from build123d import *

# Parameters (mm, degrees)
F0_W        = 130
F0_H        = 130
F1_DEPTH    = 17.5
F2_W        = 126
F2_H        = 31
F3_DEPTH    = 126
F5_W        = 122.3782406645
F5_H        = 23.2565429012
F6_DEPTH    = 7
F4_W        = 119.2743226562
F4_H        = 26.0036256061
F7_DEPTH    = 3
F8_T1_DEPTH = 50


# Not quite as in the source:
# - a fillet or chamfer that OpenCascade refuses, or shapes differently, is made with other operations: its cross-section is extruded or revolved along the edge and cut away or added


with BuildPart() as f1:
    # F0 (on Top) → F1 (new body, symmetric)
    with BuildSketch(Plane.XY):
        with Locations((2.0031377077, 1.1643140912)):
            Rectangle(F0_W, F0_H)
    extrude(amount=F1_DEPTH, both=True)

    # F2 (on face) → F3 (cut)
    with BuildSketch(Plane.XZ.offset(63.8356859088)):
        with Locations((2.0031377077, 0)):
            Rectangle(F2_W, F2_H)
    extrude(amount=-F3_DEPTH, mode=Mode.SUBTRACT)

    # F5 (on face) → F6 (cut)
    with BuildSketch(Plane(origin=(0, 66.1643140912, 0), x_dir=(-1, 0, 0), z_dir=(0, 1, 0))):
        with Locations((-2.0031377077, 0)):
            Rectangle(F5_W, F5_H)
    extrude(amount=-F6_DEPTH, mode=Mode.SUBTRACT)

    # F4 (on face) → F7 (cut)
    with BuildSketch(Plane(origin=(-62.9968622923, 0, 0), x_dir=(0, -1, 0), z_dir=(-1, 0, 0))):
        with Locations((-1.2152138836, -0.0606838628)):
            Rectangle(F4_W, F4_H)
    extrude(amount=-F7_DEPTH, mode=Mode.SUBTRACT)

    # F8: fillet of radius 3 on 4 edges, made by hand

    # F8_s2 → F8_t1 (cut)
    with BuildSketch(Plane.XY.offset(-25)):
        with BuildLine():
            add(Edge.make_bspline(
                [(-59.9968622923, 66.1643140912), (-62.9968622923, 66.1643140912), (-62.9968622923, 63.1643140912)],
                knots=[0, 0, 0, 1, 1, 1], degree=2, weights=[1, 1, 1]))
            Line((-62.9968622923, 63.1643140912), (-62.9968622923, 66.1643140912))
            Line((-62.9968622923, 66.1643140912), (-59.9968622923, 66.1643140912))
        make_face()
        with BuildLine():
            add(Edge.make_bspline(
                [(-62.9968622923, -60.8356859088), (-62.9968622923, -63.8356859088), (-59.9968622923, -63.8356859088)],
                knots=[0, 0, 0, 1, 1, 1], degree=2, weights=[1, 1, 1]))
            Line((-59.9968622923, -63.8356859088), (-62.9968622923, -63.8356859088))
            Line((-62.9968622923, -63.8356859088), (-62.9968622923, -60.8356859088))
        make_face()
        with BuildLine():
            add(Edge.make_bspline(
                [(64.0031377077, 66.1643140912), (67.0031377077, 66.1643140912), (67.0031377077, 63.1643140912)],
                knots=[0, 0, 0, 1, 1, 1], degree=2, weights=[1, 1, 1]))
            Line((67.0031377077, 63.1643140912), (67.0031377077, 66.1643140912))
            Line((67.0031377077, 66.1643140912), (64.0031377077, 66.1643140912))
        make_face()
        with BuildLine():
            add(Edge.make_bspline(
                [(67.0031377077, -60.8356859088), (67.0031377077, -63.8356859088), (64.0031377077, -63.8356859088)],
                knots=[0, 0, 0, 1, 1, 1], degree=2, weights=[1, 1, 1]))
            Line((64.0031377077, -63.8356859088), (67.0031377077, -63.8356859088))
            Line((67.0031377077, -63.8356859088), (67.0031377077, -60.8356859088))
        make_face()
    extrude(amount=F8_T1_DEPTH, mode=Mode.SUBTRACT)


solid = f1.part
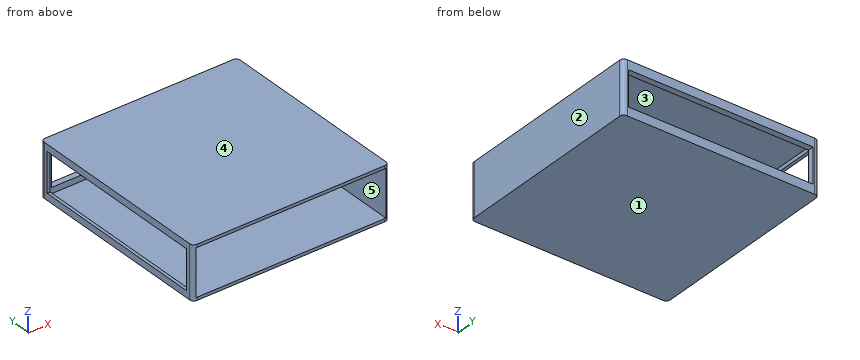
Build history of the part. All positions in model axes, mm. Face numbers are marked on the shaded views. A direction names the side the tool comes from. Round coordinates to 2 decimals unless told otherwise and drop trailing zeros. Loops run counter-clockwise (first coordinate to the right, second up) from the corner with the lowest first, then second, coordinate; pieces in that order, holes last. Notation, with made-up numbers: (67.25, 27.25) -> (108.25, 27.25) arc R19 ccw to (108.25, 44.25) -> close; hole circle Ø4 at (23, 1). An arc over 180 degrees is marked (long way). Use CSV: the item, a comma, the result in double quotes. Start each with the question number.
Q1. Saw through at A-A on x = -44. Give the cut face in (y, z).
Q2. Saw through at B-B on z = -9.5. Count the separate pieces of the cut face and the enclosed holes in it, and give its area (3 significant figures).
Q3. Mould opens along Z. For the marked faces 1, 2 and 3 say: +Z half, -Z half, draft (parallel to the pull), parting line (faces both ways), or undercut.
Q4. Which spindle directions (+Z, -Z, +X, -X, +Y, -Y) get a long thin tool onto all of the face, cutting with end or side? Do the marked faces 4 and 5. Say none if no direction does.
Q5. Drill centre lines: L1, parallel to Z at x = 4.5, y = 55.5; L2, parallel to Y at x = 33, z = 12; L3, parallel to X at y = -56.5, z = 4. Where is each one in solid material? Low to high.
Q6. Flat gauge pins, fed straight in: pin 1 Ø15.5 at (y, z) = (-29, -5) entering from -X; pin 2 Ø1 at (x, z) = (-62, -4.5) entering from +Y; pin 3 Ø0.6 at (x, z) = (-61.5, -4.5) entering from -Y; pin 4 Ø12 at (x, z) = (-22.5, 1) entering from -Y. Where does each tip first touch, or does it go through?
Q7. Saw through at C-C on y = 50.5. Give the cut face in (x, z), and give its area (3 significant figures).
Solutions:
1,outline,"(-63.84, -17.5) -> (66.16, -17.5) -> (66.16, -11.63) -> (62.16, -11.63) -> (62.16, -15.5) -> (-63.84, -15.5) -> close; (-63.84, 15.5) -> (62.16, 15.5) -> (62.16, 11.63) -> (66.16, 11.63) -> (66.16, 17.5) -> (-63.84, 17.5) -> close"
2,separate pieces,"3"
2,enclosed holes,"0"
2,area,"290 mm^2"
3,face 1,"-Z half"
3,face 2,"draft"
3,face 3,"undercut"
4,face 4,"+Z, +X, -X, +Y, -Y"
4,face 5,"-Y"
5,L1,"z = -17.5 to -15.5, 15.5 to 17.5"
5,L2,"y = 62.16 to 66.16"
5,L3,"x = 65 to 67"
6,pin 1,"stops at x = 65"
6,pin 2,"stops at y = 65.91"
6,pin 3,"stops at y = -63.68"
6,pin 4,"passes through"
7,outline,"(-63, -17.5) -> (67, -17.5) -> (67, 17.5) -> (-63, 17.5) -> (-63, 12.94) -> (-61, 12.94) -> (-61, 15.5) -> (65, 15.5) -> (65, -15.5) -> (-61, -15.5) -> (-61, -13.06) -> (-63, -13.06) -> close"
7,area,"592 mm^2"
